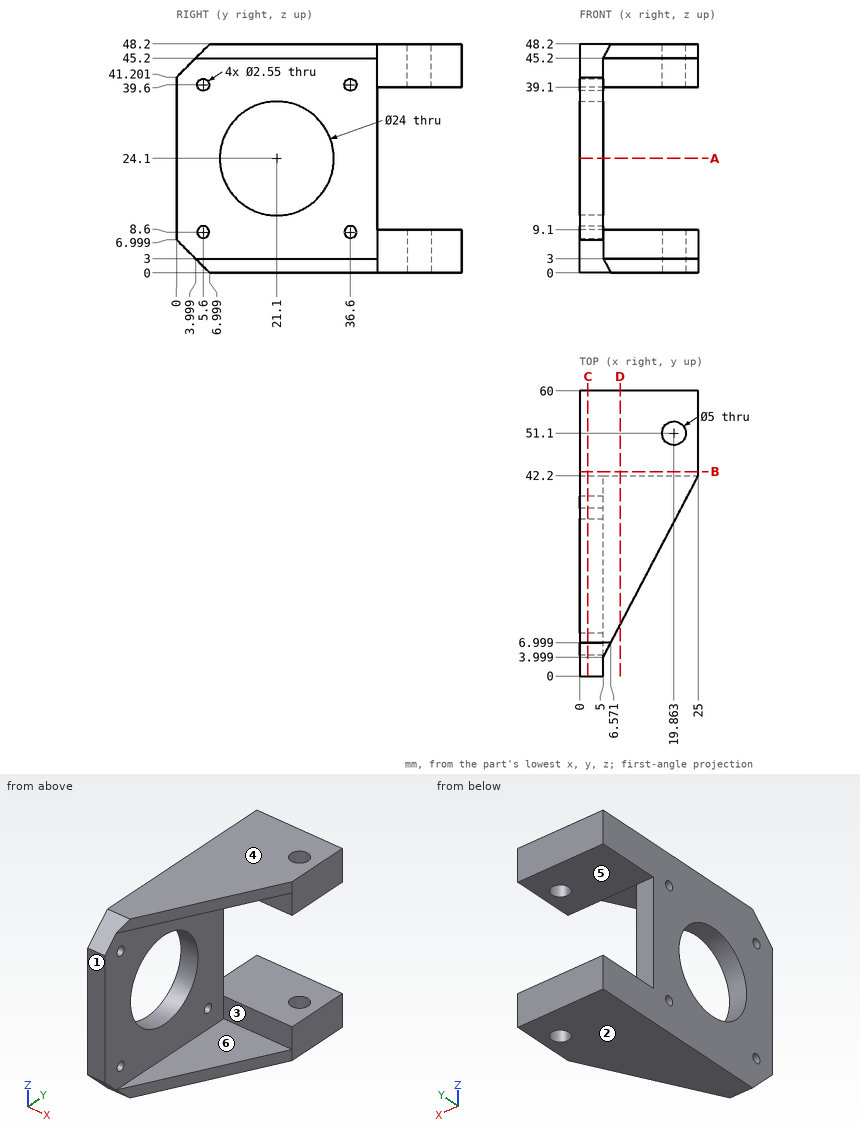
Design review of the part shown in the three views and the two pictorial views. Dimensions are in mm from the part's minimum x, y and z. A direction names the side the tool comes from. Give positions to 0.01 mm unless a question says otherwise; leave off trailing zeros. Loops run counter-clockwise (first coordinate to the right, second up) from the corner with the lowest first, then second, coordinate; pieces in that order, holes last. Notation, with made-up numbers: (-35.75, 85.5) -> (-26.75, 85.5) arc R22 ccw to (-26.75, 93.5) -> close; hole circle Ø9 at (-19, 50). An arc over 180 degrees is marked (long way). One line per item, written item: value.
Q1. We need section B-B on y = 43. Give the boundary of the cut face in (x, z), and give its area (3 significant figures).
Numbers:
outline: (0, 0) -> (25, 0) -> (25, 9.1) -> (0, 9.1) -> close; (0, 39.1) -> (25, 39.1) -> (25, 48.2) -> (0, 48.2) -> close
area: 455 mm^2
Q2. Machinability: for the marked faces 4, 5 and 6, which of the approach directions +Z, -Z, +X, -X, +Y, -Y give a long, thin tool a straight path to every point of the face, cutting with its end or side? Answer none if there is none.
Numbers:
face 4: +Z, +X, -X, +Y, -Y
face 5: +X, -X, +Y
face 6: +X, -Y
Q3. For pin 1 Ø4 at (x, y) = (19.86, 51.1) entering from +Z; pin 2 Ø3 at (y, z) = (36.6, 39.6) entering from +X; pin 3 Ø3.5 at (y, z) = (5.6, 8.6) entering from -X; pin 4 Ø6.5 at (x, z) = (16, 40.5) entering from -Y, all flat-tipped, find the tip position at first contact; note any pin that passes through.
Numbers:
pin 1: passes through
pin 2: stops at x = 5
pin 3: stops at x = 0
pin 4: stops at y = 42.2
Q4. Draft analysis for pull direction Z (two halves, no side actions). For the marked faces 1, 2 and 3, state which applies: pulls with the +Z half, pulls with the -Z half, needs draft (parallel to the pull), parting line crosses it, or undercut.
Numbers:
face 1: needs draft
face 2: pulls with the -Z half
face 3: undercut
Q5. We need section A-A on z = 24.1. Give the boundary of the cut face in (x, y).
Numbers:
outline: (0, 0) -> (5, 0) -> (5, 9.1) -> (0, 9.1) -> close; (0, 33.1) -> (5, 33.1) -> (5, 42.2) -> (0, 42.2) -> close
Q6. We need section D-D on x = 8.5. Give the boundary of the cut face in (y, z).
Numbers:
outline: (10.68, 0) -> (60, 0) -> (60, 9.1) -> (42.2, 9.1) -> (42.2, 3) -> (10.68, 3) -> close; (10.68, 45.2) -> (42.2, 45.2) -> (42.2, 39.1) -> (60, 39.1) -> (60, 48.2) -> (10.68, 48.2) -> close
Q7. For L1, parallel to Y at x = 1.8, z = 39.6 (1 decimal); L2, parallel to Z at x = 21, y = 56.5; L3, parallel to X at y = 51, z = 43 (1 decimal), list the stretches that pass through material, from the lowest coordinate up.
Numbers:
L1: y = 0 to 4.3, 6.9 to 35.3, 37.9 to 60
L2: z = 0 to 9.1, 39.1 to 48.2
L3: x = 0 to 17.4, 22.4 to 25
Q8. We need section C-C on x = 1.75. Give the number of separate pieces and of enclosed holes in the cut face, and give its area (3 significant figures).
Numbers:
separate pieces: 1
enclosed holes: 5
area: 1,840 mm^2
